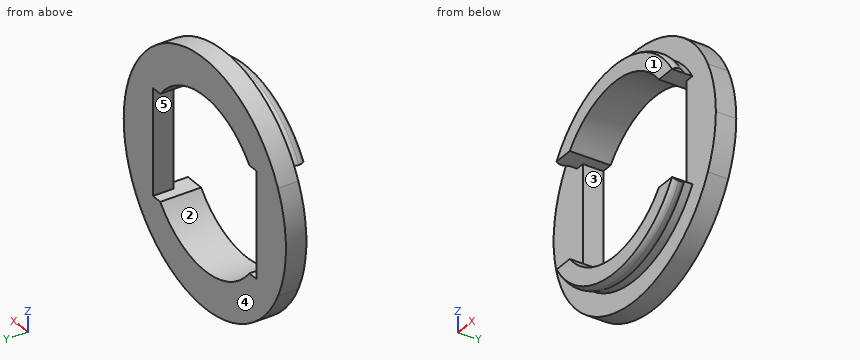
from build123d import *

# Parameters (mm, degrees)
BOSS_EXTRUDE1_DEPTH     = 2.5
BOSS_EXTRUDE2_DEPTH     = 2.5
CUT_EXTRUDE1_DEPTH      = 22.360009363
CUT_EXTRUDE1_DEPTH_BACK = 22.360009363


with BuildPart() as part:
    # Sketch1 → Boss-Extrude1 (new body)
    with BuildSketch(Plane(origin=(0, 0, 0), x_dir=(1, 0, 0), z_dir=(0, 1, 0))):
        with BuildLine():
            Line((-9.6, -6.5), (-9.6, 6.5))
            Line((-9.6, 6.5), (-13.518505835, 6.5))
            ThreePointArc((-13.518505835, 6.5), (-15, 0), (-13.518505835, -6.5))
            Line((-13.518505835, -6.5), (-9.6, -6.5))
        make_face()
        with BuildLine():
            Line((9.6, -6.5), (-9.6, -6.5))
            Line((-9.6, -6.5), (-13.518505835, -6.5))
            ThreePointArc((-13.518505835, -6.5), (0, -15), (13.518505835, -6.5))
            Line((13.518505835, -6.5), (9.6, -6.5))
        make_face()
        with BuildLine():
            Line((-13.518505835, 6.5), (-9.6, 6.5))
            Line((-9.6, 6.5), (9.6, 6.5))
            Line((9.6, 6.5), (13.518505835, 6.5))
            ThreePointArc((13.518505835, 6.5), (0, 15), (-13.518505835, 6.5))
        make_face()
        with BuildLine():
            Line((13.518505835, 6.5), (9.6, 6.5))
            Line((9.6, 6.5), (9.6, -6.5))
            Line((9.6, -6.5), (13.518505835, -6.5))
            ThreePointArc((13.518505835, -6.5), (14.624937393, -3.333347603), (15, 0))
            ThreePointArc((15, 0), (14.624937393, 3.333347603), (13.518505835, 6.5))
        make_face()
    extrude(amount=BOSS_EXTRUDE1_DEPTH)

    # Sketch2 → Boss-Extrude2 (add)
    with BuildSketch(Plane.XZ):
        with BuildLine():
            ThreePointArc((10.677078252, 6.5), (0, 12.5), (-10.677078252, 6.5))
            Line((-10.677078252, 6.5), (-9.6, 6.5))
            Line((-9.6, 6.5), (-8.246211251, 6.5))
            ThreePointArc((-8.246211251, 6.5), (0, 10.5), (8.246211251, 6.5))
            Line((8.246211251, 6.5), (9.6, 6.5))
            Line((9.6, 6.5), (10.677078252, 6.5))
        make_face()
        with BuildLine():
            Line((-9.6, -6.5), (-10.677078252, -6.5))
            ThreePointArc((-10.677078252, -6.5), (0, -12.5), (10.677078252, -6.5))
            Line((10.677078252, -6.5), (9.6, -6.5))
            Line((9.6, -6.5), (8.246211251, -6.5))
            ThreePointArc((8.246211251, -6.5), (0, -10.5), (-8.246211251, -6.5))
            Line((-8.246211251, -6.5), (-9.6, -6.5))
        make_face()
    extrude(amount=BOSS_EXTRUDE2_DEPTH)

    # Sketch2_3 → Cut-Extrude1 (cut, two sides)
    with BuildSketch(Plane.XZ) as cut_extrude1_sk:
        with BuildLine():
            ThreePointArc((8.246211251, 6.5), (0, 10.5), (-8.246211251, 6.5))
            Line((-8.246211251, 6.5), (8.246211251, 6.5))
        make_face()
        with BuildLine():
            Line((8.246211251, -6.5), (-8.246211251, -6.5))
            ThreePointArc((-8.246211251, -6.5), (0, -10.5), (8.246211251, -6.5))
        make_face()
    extrude(amount=CUT_EXTRUDE1_DEPTH, mode=Mode.SUBTRACT)
    extrude(cut_extrude1_sk.sketch, amount=-CUT_EXTRUDE1_DEPTH_BACK, mode=Mode.SUBTRACT)

    # Sweep2: sweep along a curve in space
    with BuildLine() as sweep2_path:
        ThreePointArc((10.677078252, -2.5, 6.5), (0, -2.5, 12.5), (-10.677078252, -2.5, 6.5))
    # Sketch4 → Sweep2 (sweep)
    with BuildSketch(Plane(origin=(0, 0, 6.5), x_dir=(-1, 0, 0), z_dir=(0, 0, -1))):
        with BuildLine():
            Line((10.677078252, -2.5), (10.677078252, -1))
            ThreePointArc((10.677078252, -1), (10.899296653, -1.346112639), (10.977078252, -1.75))
            ThreePointArc((10.977078252, -1.75), (10.899296653, -2.153887361), (10.677078252, -2.5))
        make_face()
    sweep(path=sweep2_path.line)

    # Sweep4: sweep along a curve in space
    with BuildLine() as sweep4_path:
        ThreePointArc((-10.677078252, -2.5, -6.5), (0, -2.5, -12.5), (10.677078252, -2.5, -6.5))
    # Sketch11 → Sweep4 (sweep)
    with BuildSketch(Plane.XY.offset(-6.5)):
        with BuildLine():
            Line((-10.677078252, -2.5), (-10.677078252, -1))
            ThreePointArc((-10.677078252, -1), (-10.899296653, -1.346112639), (-10.977078252, -1.75))
            ThreePointArc((-10.977078252, -1.75), (-10.899296653, -2.153887361), (-10.677078252, -2.5))
        make_face()
    sweep(path=sweep4_path.line)


solid = part.part
Could you check a few things on this model? Use its own coordinates, in mm. Face numbers are marked on the shaded views. A direction names the side the tool comes from. Give positions to 0.01 mm unless a question says otherwise; leave off trailing zeros. Write each loop counter-clockwise with the first axis right and the second up, starting at its lowest first coordinate (ties: lowest second). Pieces come first, ordered by that corner, then holes. Notation, with made-up numbers: (-6, -37.75) - (31, -37.75) arc R37 ccw to (31, -0.75) - close; hole circle Ø10 at (41.5, -3.75). An arc over 180 degrees is marked (long way). Use CSV: the item, a comma, the result in double quotes. Start each with the question number.
Item 1: If we mould it in two halves opening along Z, with no side actions, what happens to the marked faces 1, 2 and 3? For each: pulls with the +Z half, pulls with the -Z half, needs draft (parallel to the pull), parting line crosses it, or undercut.
Item 2: For the marked faces 4 and 5, which set-ups out of +Z, -Z, +X, -X, +Y, -Y let a thin tool reach every point of the face, with its end or its side?
Item 3: I want a section at D-D, the plane x = 11.75. Please give me the cut outline in (y, z).
Item 4: I'm going to push flat-ended pins straight in: pin 1 (1 mm diameter, centred on x = 7, z = -11, fed in from -Y); pin 2 (3 mm diameter, centred on x = 4.5, y = 1.5, fed in from +Z); pin 3 (1.5 mm diameter, centred on x = 8.5, y = 0, fed in from -Z). Where does each tip first touch, or does it pass through?
Item 5: I want a section at C-C, the plane z = -6. Please give me the cut outline in (x, y), then the cut area to 3 significant figures.
Item 6: I want a section at A-A, the plane y = 1.3. Please give me the cut outline in (x, z).
Item 7: If I drill on line 1 along Z through (x, y) = (0, 0.9); line 2 along Y through (x, z) = (9.75, -9.5); line 3 along Z through (x, y) = (-4.75, 0.7), over which ranges is the centre line in solid material (lowest first)?
Item 8: I want a section at B-B, the plane z = 1. Please give me the cut outline in (x, y), then the cut area to 3 significant figures.
Findings:
1,face 1,"needs draft"
1,face 2,"undercut"
1,face 3,"undercut"
2,face 4,"+Z, -Z, +X, -X, +Y"
2,face 5,"+Y, -Y"
3,outline,"(0, -9.32) - (2.5, -9.32) - (2.5, 9.32) - (0, 9.32) - close"
4,pin 1,"stops at y = -2.45"
4,pin 2,"stops at z = 14.7"
4,pin 3,"stops at z = -12.84"
5,outline,"(-13.75, 0) - (-9.6, 0) - (-9.6, 2.5) - (-13.75, 2.5) - close; (9.6, 0) - (13.75, 0) - (13.75, 2.5) - (9.6, 2.5) - close"
5,area,"20.7 mm2"
6,outline,"circle Ø30 at (0, 0); hole (-9.6, -6.5) - (-8.25, -6.5) arc R10.5 ccw to (8.25, -6.5) - (9.6, -6.5) - (9.6, 6.5) - (8.25, 6.5) arc R10.5 ccw to (-8.25, 6.5) - (-9.6, 6.5) - close"
7,line 1,"z = -15 to -10.5, 10.5 to 15"
7,line 2,"y = 0 to 2.5"
7,line 3,"z = -14.23 to -9.36, 9.36 to 14.23"
8,outline,"(-14.97, 0) - (-9.6, 0) - (-9.6, 2.5) - (-14.97, 2.5) - close; (9.6, 0) - (14.97, 0) - (14.97, 2.5) - (9.6, 2.5) - close"
8,area,"26.8 mm2"
